from build123d import *

# Parameters (mm, degrees)
SKETCH1_R           = 5.5
BOSS_EXTRUDE1_DEPTH = 40
SKETCH2_R           = 2
CUT_EXTRUDE1_DEPTH  = 41
FILLET1_R           = 0.5


with BuildPart() as part:
    # Sketch1 → Boss-Extrude1 (new body)
    with BuildSketch(Plane.XY):
        Circle(SKETCH1_R)
    extrude(amount=BOSS_EXTRUDE1_DEPTH)

    # Sketch2 → Cut-Extrude1 (cut, through all)
    with BuildSketch(Plane.XY.offset(40)):
        Circle(SKETCH2_R)
    extrude(amount=-CUT_EXTRUDE1_DEPTH, mode=Mode.SUBTRACT)

    # Fillet1
    fillet1_edges = [part.edges().sort_by_distance(p)[0] for p in [
        (-5.5, 0, 0),
        (-5.5, 0, 40),
        (-2, 0, 0),
        (-2, 0, 40),
    ]]
    fillet(fillet1_edges, radius=FILLET1_R)


solid = part.part
Work out the finished part from the listing and answer in its coordinate system (mm). Round coordinates to 2 decimals unless told otherwise and drop trailing zeros. Order: outer loops, then holes, each group sorted by start corner. A loop starts at its lowest first (then second) coordinate and runs counter-clockwise, first axis right, second up. Notation, with made-up numbers: M -6,82 L 52,82 A10 ccw 52,98 Z; hole C -8.5,14.5 d3. An arc over 180 degrees is marked long. Put each result on its own line as item: value. Start each with the question number.
Q1. For a pull along X with two mould halves and no side action, classify faces 1 (the cylindrical face through (0, -2, 20)), 2 (the flat face through (2, -2, 40)), 3 (the cylindrical face through (-1.19, -5.37, 19.73)) as pulls with the +X half, pulls with the -X half, needs draft (parallel to the pull), parting line crosses it, or undercut.
Q2. Section C-C, the plane z = 13 is taken. Write down the section's boundary in (x, y).
Q3. Section A-A, the plane y = 0 is taken. Write down the section's boundary in (x, z).
Q4. A flat-ended cylindrical pin translates along its axis: pin 1 (2 mm diameter, centred on x = -3, z = 19.5, fed in from +Y). Find the tip coordinate at first contact, or state that the pin passes through.
Q5. Straight lines are drawn through the part: L1, parallel to Y at x = 0, z = 31; L2, parallel to Y at x = 1.25, z = 33.5; L3, parallel to Z at x = -2.25, y = 1. For each, find the intervals that lie inside material, in ascending order. Write a range as [from, to].
Findings below:
1. face 1: undercut
1. face 2: needs draft
1. face 3: parting line crosses it
2. outline: C 0,0 d11; hole C 0,0 d4
3. outline: M -5.5,0.5 A0.5 ccw -5,0 L -2.5,0 A0.5 ccw -2,0.5 L -2,39.5 A0.5 ccw -2.5,40 L -5,40 A0.5 ccw -5.5,39.5 Z; M 2,0.5 A0.5 ccw 2.5,0 L 5,0 A0.5 ccw 5.5,0.5 L 5.5,39.5 A0.5 ccw 5,40 L 2.5,40 A0.5 ccw 2,39.5 Z
4. pin 1: stops at y = 5.12
5. L1: y = [-5.5, -2], [2, 5.5]
5. L2: y = [-5.36, -1.56], [1.56, 5.36]
5. L3: z = [0, 40]
